Autodesk Fusion 360 part; units mm, degrees
sketch "Esquisse1" plane through (0, 0, 0) normal (0, 1, 0) x (1, 0, 0)
sketch "Esquisse2" plane through (0, 0, 0) normal (0, 1, 0) x (1, 0, 0)
  line L0 (-7.1984, 5.7929) -> (5.54, 13.0097)
  line L1 (12.224, 8.699) -> (12.1271, -9.222)
  line L2 (5.2978, -12.903) -> (-5.0189, -7.0424)
  line L3 (-5.0189, -7.0424) -> (-4.4376, -10.7234)
  line L4 (-5.9876, -11.014) -> (-6.8594, -5.9768)
  line L5 (-6.8594, -5.9768) -> (-10.3467, -3.8457)
  line L6 (-10.6857, 3.807) -> (-8.6999, 5.0179)
  line L7 (-8.6999, 5.0179) -> (-9.6202, 10.0067)
  line L8 (-7.1984, 5.7929) -> (-8.0703, 10.2973)
  line L9 (-8.6999, 5.0179) -> (-7.1984, 5.7929)
  line L10 (-6.8594, -5.9768) -> (-5.0189, -7.0424)
  line L11 (-5.0189, -7.0424) -> (-5.4827, -4.0424)
  line L12 (-6.8594, -5.9768) -> (-7.1185, -4.1951)
  line L13 (-8.6999, 5.0179) -> (-7.7946, -0.5527)
  line L14 (-7.1984, 5.7929) -> (-6.2024, -0.2692)
  spline S0 degree 5 poles (-10.6857, 3.807) (-10.7699, 3.7194) (-10.9329, 3.5405) (-11.1609, 3.262) (-11.4318, 2.8699) (-11.7139, 2.345) (-11.9372, 1.7861) (-12.0992, 1.1967) (-12.1982, 0.5832) (-12.2336, -0.0425) (-12.2055, -0.6652) (-12.1151, -1.2686) (-11.9635, -1.8369) (-11.7524, -2.3571) (-11.4841, -2.8215) (-11.1611, -3.227) (-10.8608, -3.5037) (-10.6126, -3.6849) (-10.437, -3.794) (-10.3467, -3.8457) knots 0 0 0 0 0 0 0.066667 0.133333 0.2 0.266667 0.333333 0.4 0.466667 0.533333 0.6 0.666667 0.733333 0.8 0.866667 0.933333 1 1 1 1 1 1
  spline S1 degree 5 poles (-5.9876, -11.014) (-5.98, -11.0815) (-5.962, -11.211) (-5.9262, -11.389) (-5.8609, -11.5936) (-5.7497, -11.7934) (-5.6098, -11.9361) (-5.4437, -12.0212) (-5.2571, -12.05) (-5.0595, -12.0267) (-4.8639, -11.9579) (-4.6838, -11.8508) (-4.5321, -11.7128) (-4.4193, -11.5504) (-4.3509, -11.3682) (-4.3292, -11.1692) (-4.3494, -10.998) (-4.3855, -10.8632) (-4.4187, -10.7705) (-4.4376, -10.7234) knots 0 0 0 0 0 0 0.066667 0.133333 0.2 0.266667 0.333333 0.4 0.466667 0.533333 0.6 0.666667 0.733333 0.8 0.866667 0.933333 1 1 1 1 1 1
  spline S2 degree 5 poles (-9.6202, 10.0067) (-9.6184, 10.0519) (-9.6131, 10.1401) (-9.5997, 10.2658) (-9.5709, 10.4199) (-9.5164, 10.5894) (-9.4434, 10.7347) (-9.3521, 10.854) (-9.2441, 10.9456) (-9.1223, 11.0075) (-8.9906, 11.0379) (-8.8533, 11.0351) (-8.7144, 10.9979) (-8.577, 10.9258) (-8.443, 10.8194) (-8.3135, 10.6798) (-8.2137, 10.5424) (-8.1411, 10.4253) (-8.0937, 10.341) (-8.0703, 10.2973) knots 0 0 0 0 0 0 0.066667 0.133333 0.2 0.266667 0.333333 0.4 0.466667 0.533333 0.6 0.666667 0.733333 0.8 0.866667 0.933333 1 1 1 1 1 1
  spline S3 degree 5 poles (-7.7946, -0.5527) (-7.7612, -0.6069) (-7.6946, -0.7105) (-7.595, -0.8519) (-7.463, -1.012) (-7.2995, -1.1638) (-7.138, -1.2662) (-6.9798, -1.3193) (-6.8266, -1.3244) (-6.6815, -1.2859) (-6.5481, -1.2112) (-6.4304, -1.1085) (-6.3323, -0.9864) (-6.2568, -0.8522) (-6.2053, -0.7111) (-6.1784, -0.5661) (-6.1761, -0.4483) (-6.1851, -0.359) (-6.1959, -0.2992) (-6.2024, -0.2692) knots 0 0 0 0 0 0 0.066667 0.133333 0.2 0.266667 0.333333 0.4 0.466667 0.533333 0.6 0.666667 0.733333 0.8 0.866667 0.933333 1 1 1 1 1 1
  spline S4 degree 5 poles (-7.1185, -4.1951) (-7.1273, -4.1462) (-7.1416, -4.0505) (-7.1525, -3.9136) (-7.1458, -3.7446) (-7.1017, -3.5566) (-7.0219, -3.3935) (-6.9082, -3.2574) (-6.7647, -3.1513) (-6.5991, -3.0788) (-6.421, -3.0438) (-6.2407, -3.0501) (-6.0678, -3.1006) (-5.9095, -3.1972) (-5.77, -3.3397) (-5.6512, -3.5272) (-5.5732, -3.712) (-5.5243, -3.8698) (-5.4958, -3.9835) (-5.4827, -4.0424) knots 0 0 0 0 0 0 0.066667 0.133333 0.2 0.266667 0.333333 0.4 0.466667 0.533333 0.6 0.666667 0.733333 0.8 0.866667 0.933333 1 1 1 1 1 1
  spline S5 degree 5 poles (5.54, 13.0097) (5.6415, 13.057) (5.8467, 13.1442) (6.1609, 13.2531) (6.5927, 13.3541) (7.1534, 13.4049) (7.733, 13.3783) (8.3266, 13.273) (8.925, 13.0897) (9.5138, 12.8319) (10.0763, 12.5047) (10.5954, 12.1138) (11.0555, 11.665) (11.4452, 11.1636) (11.7593, 10.6142) (11.9964, 10.0205) (12.1249, 9.512) (12.1875, 9.1125) (12.2143, 8.8382) (12.224, 8.699) knots 0 0 0 0 0 0 0.066667 0.133333 0.2 0.266667 0.333333 0.4 0.466667 0.533333 0.6 0.666667 0.733333 0.8 0.866667 0.933333 1 1 1 1 1 1
  spline S6 degree 5 poles (12.1271, -9.222) (12.1122, -9.3477) (12.0761, -9.5956) (12.0029, -9.957) (11.8667, -10.4177) (11.6309, -10.9569) (11.3289, -11.4568) (10.961, -11.9136) (10.5308, -12.3221) (10.0458, -12.6759) (9.5162, -12.9679) (8.9528, -13.1911) (8.3662, -13.3397) (7.7651, -13.4101) (7.155, -13.4017) (6.5396, -13.3162) (6.0444, -13.1875) (5.6716, -13.058) (5.4225, -12.9571) (5.2978, -12.903) knots 0 0 0 0 0 0 0.066667 0.133333 0.2 0.266667 0.333333 0.4 0.466667 0.533333 0.6 0.666667 0.733333 0.8 0.866667 0.933333 1 1 1 1 1 1
  line L15 (-5.7636, 8.9045) -> (-6.1644, 10.9757)
  spline S7 degree 3 poles (-11.6273, 9.8625) (-11.6244, 9.9366) (-11.6215, 10.0106) (-11.6187, 10.0847) (-11.5981, 10.6109) (-11.5086, 11.1908) (-11.1328, 11.7914) (-10.8094, 12.3082) (-10.2251, 12.7973) (-9.519, 12.9643) (-8.8485, 13.1228) (-8.1086, 12.9653) (-7.5907, 12.6581) (-6.9707, 12.2904) (-6.6308, 11.8133) (-6.3692, 11.3538) (-6.3483, 11.3172) (-6.328, 11.2804) (-6.3082, 11.2434) (-6.2603, 11.1542) (-6.2124, 11.065) (-6.1644, 10.9757) knots -0.065512 -0.065512 -0.065512 -0.065512 0 0 0 0.267845 0.267845 0.267845 0.498306 0.498306 0.498306 0.717136 0.717136 0.717136 0.979101 0.979101 0.979101 1 1 1 1.081691 1.081691 1.081691 1.081691
  line L16 (-10.9165, 6.0088) -> (-11.6273, 9.8625)
  line L17 (-11.9486, 5.3795) -> (-10.9165, 6.0088)
  spline S8 degree 3 poles (-11.9486, 5.3795) (-12.0085, 5.3171) (-12.0684, 5.2547) (-12.1284, 5.1923) (-13.1498, 4.1285) (-13.8529, 2.7498) (-14.1047, 1.2701) (-14.3725, -0.3036) (-14.196, -1.9549) (-13.4657, -3.359) (-12.9883, -4.2766) (-12.2497, -5.0545) (-11.3675, -5.5657) knots -0.028469 -0.028469 -0.028469 -0.028469 0 0 0 0.361544 0.361544 0.361544 0.746051 0.746051 0.746051 0.997343 0.997343 0.997343 0.997343
  line L18 (-8.6755, -7.2108) -> (-11.3675, -5.5657)
  line L19 (-7.9672, -11.3033) -> (-8.6755, -7.2108)
  spline S9 degree 3 poles (-7.9672, -11.3033) (-7.9089, -11.7699) (-7.8016, -12.2574) (-7.48, -12.777) (-7.2137, -13.2071) (-6.7471, -13.6451) (-6.1942, -13.8602) (-5.5957, -14.0931) (-4.9994, -14.068) (-4.525, -13.9431) (-3.8951, -13.7771) (-3.3791, -13.4541) (-2.9579, -12.9299) (-2.5662, -12.4424) (-2.3301, -11.744) (-2.3414, -11.1207) (-2.343, -11.0299) (-2.3489, -10.9406) (-2.3583, -10.854) knots 0.008172 0.008172 0.008172 0.008172 0.179714 0.179714 0.179714 0.321692 0.321692 0.321692 0.475411 0.475411 0.475411 0.679585 0.679585 0.679585 0.869444 0.869444 0.869444 0.897086 0.897086 0.897086 0.897086
  line L20 (4.4033, -14.6951) -> (-2.3583, -10.854)
  spline S10 degree 3 poles (14.1265, -9.3452) (14.1221, -9.3824) (14.1177, -9.4196) (14.1133, -9.4569) (13.9484, -10.8507) (13.3861, -12.1991) (12.4284, -13.2435) (11.2723, -14.5046) (9.608, -15.2956) (7.8758, -15.3872) (6.7194, -15.4484) (5.5728, -15.2024) (4.5018, -14.7378) (4.469, -14.7236) (4.4361, -14.7093) (4.4033, -14.6951) knots -0.011842 -0.011842 -0.011842 -0.011842 0 0 0 0.331858 0.331858 0.331858 0.732526 0.732526 0.732526 1 1 1 1.010536 1.010536 1.010536 1.010536
  line L21 (14.2244, 8.7631) -> (14.1265, -9.3452)
  spline S11 degree 3 poles (4.6236, 14.7892) (4.6477, 14.8004) (4.6718, 14.8116) (4.696, 14.8229) (5.9988, 15.4293) (7.5313, 15.5394) (8.9662, 15.1545) (10.3979, 14.7705) (11.7739, 13.9432) (12.7601, 12.7117) (13.6356, 11.6185) (14.1212, 10.2454) (14.2192, 8.8378) (14.2209, 8.8129) (14.2226, 8.788) (14.2244, 8.7631) knots -0.009504 -0.009504 -0.009504 -0.009504 0 0 0 0.346802 0.346802 0.346802 0.692835 0.692835 0.692835 1 1 1 1.007161 1.007161 1.007161 1.007161
  line L22 (-5.7636, 8.9045) -> (4.6236, 14.7892)
  point P0 (-12.1008, 1.1081)
  point P1 (-11.8883, -1.9946)
  point P2 (-5.4039, -12.0173)
  point P3 (-4.534, -11.6977)
  point P4 (-9.3358, 10.8596)
  point P5 (-8.7483, 11.0014)
  point P6 (-6.9047, -1.3161)
  point P7 (-6.3172, -0.9514)
  point P8 (-6.9028, -3.2668)
  point P9 (-6.1132, -3.0951)
  point P10 (8.1681, 13.2894)
  point P11 (10.9712, 11.7249)
  point P12 (10.9712, -11.8733)
  point P13 (8.4289, -13.3075)
  dimension "d3" = -2
extrude "Extrusion1" add sketch "Esquisse2" along normal blind 1 contours L7 L8 L9 S2 | L0 L1 L2 L5 L6 L11 L12 L13 L14 S0 S3 S4 S5 S6 | L3 L4 L10 S1 makes body 1 at (6.2735, 0, 1.4601)
extrude "Extrusion2" add sketch "Esquisse2" against normal blind 1 separate body contours L7 L8 L9 S2 | L9 L13 L14 S3 | L0 L1 L2 L5 L6 L11 L12 L13 L14 S0 S3 S4 S5 S6 | L3 L4 L10 S1 | L10 L11 L12 S4 | L15 S7 L16 L17 S8 L18 L19 S9 L20 S10 L21 S11 L22 makes body 2
combine "Combiner1" operation add target body 2 tool bodies 1
Input: part model. Units: mm. Frame: model coordinates. A direction names the side the tool comes from. Coordinates: 2 decimals unless noted, no trailing zeros. Answer as a JSON object with one key per item and string values.
1. First-contact query: P1, Ø1.7, axis at x = -6, z = 4.5, coming from the +Y side. Flat tip, straight axial feed; report the tip coordinate or a pass-through.
Result set:
{"P1": "stops at y = 1"}
2. Mould query, pull axis X, two halves, no side actions, for faces 1 (the face through (-6.707, 0.493, -2.804)), 2 (the face through (-9.154, 0.493, -7.477)), 3 (the face through (-2, 0, 9)), 4 (the face through (-6, 1, 9)). Classes: released by +X, released by -X, zero draft, split by the parting line, or undercut.
Result set:
{"face 1": "undercut", "face 2": "released by -X", "face 3": "undercut", "face 4": "zero draft"}
3. Access query for faces 5 (the face through (-9.71, 0.49, -4.4)), 6 (the face through (-5.25, 0.49, 5.56)), 7 (the face through (-11.267, -0.493, -7.909)), 8 (the face through (-6.417, 0.493, 8.531)). Directions: +Z, -Z, +X, -X, +Y, -Y. A direction counts if a zero-diameter tool reaches every point of the face in a straight line with its end or side. Return the directions, or none.
Result set:
{"face 5": "-X, +Y", "face 6": "+Y", "face 7": "-X, +Y, -Y", "face 8": "+Z, -X, +Y"}
4. Material intervals for line 1 (X direction, y = 0.4, z = -1); line 2 (Y direction, x = 3, z = -12.5); line 3 (X direction, y = -0.8, z = 12.5), sorted ascending. Write a range as from..to.
Result set:
{"line 1": "x = -12.12..-8.05, -6.41..12.18", "line 2": "y = -1..0", "line 3": "x = -7.63..-2.68, 0.54..13.01"}
